Design review of the part shown in the three views and the two pictorial views. Dimensions are in mm from the part's minimum x, y and z. A direction names the side the tool comes from. Coordinates: 2 decimals unless noted, no trailing zeros. Loops run counter-clockwise (first coordinate to the right, second up) from the corner with the lowest first, then second, coordinate; pieces in that order, holes last. Notation, with made-up numbers: (69, 51) -> (84, 51) arc R21 ccw to (84, 79) -> close; hole circle Ø3 at (7, 51). An arc over 180 degrees is marked (long way). Answer in a Markdown table with one row per item.
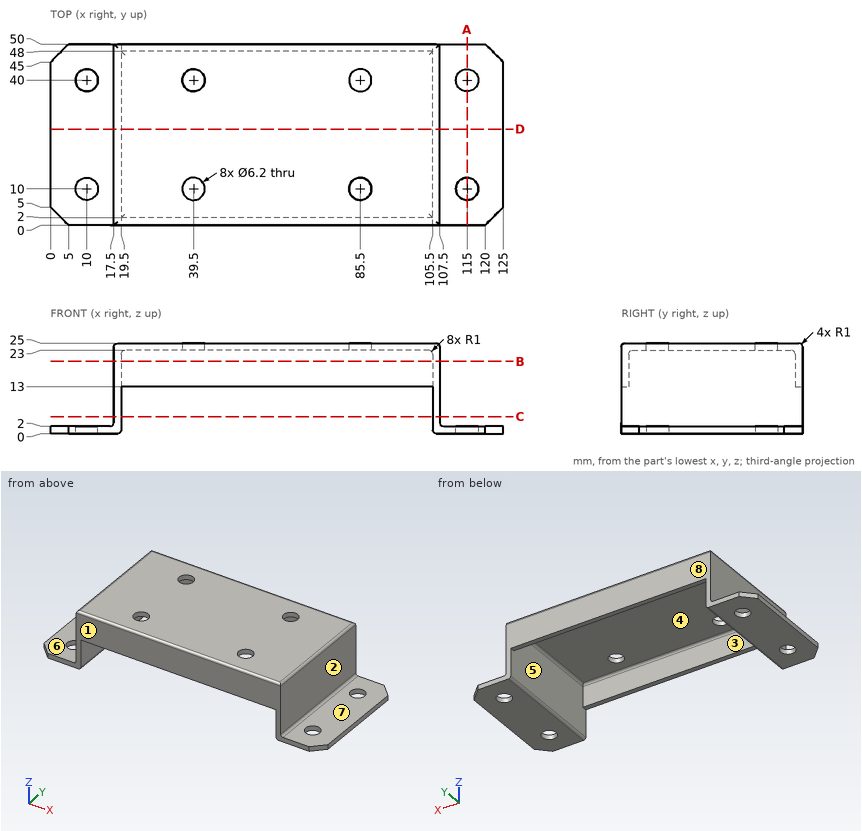
(1) Take a section at A-A on x = 115. Give the boundary of the cut face in (y, z).
Evaluation:
| item | result |
|---|---|
| outline | (0, 0) -> (6.9, 0) -> (6.9, 2) -> (0, 2) -> close; (13.1, 0) -> (36.9, 0) -> (36.9, 2) -> (13.1, 2) -> close; (43.1, 0) -> (50, 0) -> (50, 2) -> (43.1, 2) -> close |
(2) Tool access review of the marked faces 5, 6, 7 and 8: name each direction out of +Z, -Z, +X, -X, +Y, -Y from which nothing blocks a thin tool from reaching the whole face with its end or side.
Evaluation:
| item | result |
|---|---|
| face 5 | -Z |
| face 6 | +Z, -X, +Y, -Y |
| face 7 | +Z, +X, +Y, -Y |
| face 8 | +Z, -Z, +X, -X, +Y |
(3) For pin 1 (2 mm diameter, centred on x = 57, y = 1, fed in from -Z); pin 2 (10 mm diameter, centred on x = 39.5, y = 10, fed in from -Z); pin 3 (10 mm diameter, centred on y = 13, z = 16.5, fed in from +X); pin 4 (10 mm diameter, centred on x = 71.5, z = 18.5, fed in from -Y), all flat-tipped, find the tip position at first contact; note any pin that passes through.
Evaluation:
| item | result |
|---|---|
| pin 1 | stops at z = 13 |
| pin 2 | stops at z = 23 |
| pin 3 | stops at x = 107.5 |
| pin 4 | stops at y = 0 |
(4) Draft analysis for pull direction X (two halves, no side actions). For the marked faces 1, 2, 3 and 4, state which applies: pulls with the +X half, pulls with the -X half, needs draft (parallel to the pull), parting line crosses it, or undercut.
Evaluation:
| item | result |
|---|---|
| face 1 | needs draft |
| face 2 | pulls with the +X half |
| face 3 | undercut |
| face 4 | undercut |
(5) Take a section at D-D on y = 26.5. Give the boundary of the cut face in (x, z).
Evaluation:
| item | result |
|---|---|
| outline | (0, 0) -> (18.5, 0) arc R1 ccw to (19.5, 1) -> (19.5, 22) arc R1 cw to (20.5, 23) -> (104.5, 23) arc R1 cw to (105.5, 22) -> (105.5, 1) arc R1 ccw to (106.5, 0) -> (125, 0) -> (125, 2) -> (108.5, 2) arc R1 cw to (107.5, 3) -> (107.5, 24) arc R1 ccw to (106.5, 25) -> (18.5, 25) arc R1 ccw to (17.5, 24) -> (17.5, 3) arc R1 cw to (16.5, 2) -> (0, 2) -> close |
(6) Take a section at C-C on z = 4.75. Give the boundary of the cut face in (x, y).
Evaluation:
| item | result |
|---|---|
| outline | (17.5, 0) -> (19.5, 0) -> (19.5, 50) -> (17.5, 50) -> close; (105.5, 0) -> (107.5, 0) -> (107.5, 50) -> (105.5, 50) -> close |
(7) To check wall thickness, follow probe 1 along Y at (x, z) = (10, 0.85); probe 2 along Y at (x, z) = (83, 17); probe 3 along X at (y, z) = (45, 14). State the ranges of each line that lie inside material, in increasing order.
Evaluation:
| item | result |
|---|---|
| probe 1 | y = 0 to 6.9, 13.1 to 36.9, 43.1 to 50 |
| probe 2 | y = 0 to 2, 48 to 50 |
| probe 3 | x = 17.5 to 19.5, 105.5 to 107.5 |
(8) Take a section at B-B on z = 20. Give the boundary of the cut face in (x, y).
Evaluation:
| item | result |
|---|---|
| outline | (17.5, 0) -> (107.5, 0) -> (107.5, 50) -> (17.5, 50) -> close; hole (19.5, 2) -> (105.5, 2) -> (105.5, 48) -> (19.5, 48) -> close |
